The model under review builds one solid part; all positions refer to its coordinate system, in mm. Give positions to 0.01 mm unless a question says otherwise; leave off trailing zeros. Loops run counter-clockwise (first coordinate to the right, second up) from the corner with the lowest first, then second, coordinate; pieces in that order, holes last. Notation, with made-up numbers: M 15,67 L 48,67 A27 cw 48,104 Z; hole C 24,6 d5. An arc over 180 degrees is marked long. Write item = value, one per line. Start each with the question number.
1. For pin 1 (10 mm diameter, centred on y = -126.5, z = 7, fed in from +X); pin 2 (1 mm diameter, centred on y = 130.5, z = 10.5, fed in from +X), all flat-tipped, find the tip position at first contact; note any pin that passes through.
2. We need section A-A on x = -21. Give the boundary of the cut face in (y, z), then the cut area to 3 significant figures.
3. Wall thickness on line 1 along Y through (x, z) = (41, 5); line 2 along X through (y, z) = (125, 12.75); line 3 along X through (y, z) = (146.5, 17.5): over which ranges is each line inside the solid? List them lowest first. Write a range as from..to.
4. We need section C-C on z = 5.75. Give the boundary of the cut face in (x, y).
5. We need section D-D on x = 169. Give the boundary of the cut face in (y, z), then the cut area to 3 significant figures.
6. We need section B-B on y = 136.5. Give the boundary of the cut face in (x, z), then the cut area to 3 significant figures.
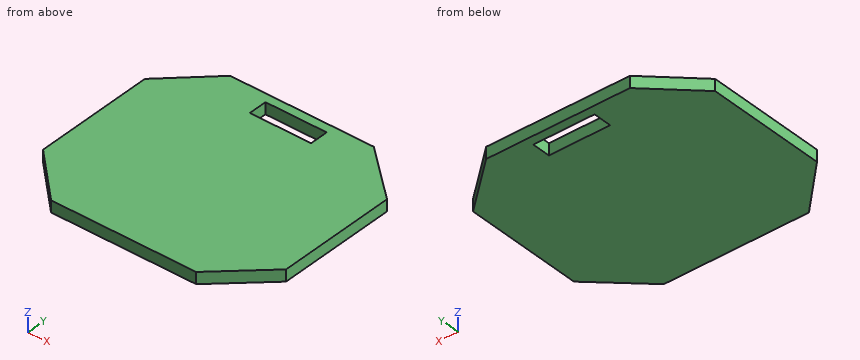
from build123d import *

# Parameters (mm, degrees)
F0_W     = 400
F0_H     = 350
F1_DEPTH = 19
F3_DEPTH = 19.001
F5_DEPTH = 19.001


with BuildPart() as f1:
    # F0 (on Top) → F1 (new body)
    with BuildSketch(Plane.XY):
        Rectangle(F0_W, F0_H)
    extrude(amount=F1_DEPTH)

    # F2 (on face) → F3 (cut, through all)
    with BuildSketch(Plane.XY.offset(19)):
        Polygon((-200, 175), (-200, 100.611582), (-122.030288, 175), align=None)
        Polygon((200, 175), (114.702843, 175), (200, 99.48428), align=None)
        Polygon((200, -97.793318), (116.957434, -175), (200, -175), align=None)
        Polygon((-122.030288, -175), (-200, -98.356977), (-200, -175), align=None)
    extrude(amount=-F3_DEPTH, mode=Mode.SUBTRACT)

    # F4 (on face) → F5 (cut, through all)
    with BuildSketch(Plane.XY.offset(19)):
        Polygon((-51.574003, 160.358503), (-51.574003, 129.921392), (49.319401, 129.921392), (49.319401, 160.358503), (39.737348, 160.358503), align=None)
    extrude(amount=-F5_DEPTH, mode=Mode.SUBTRACT)


solid = f1.part
Final values:
q1.pin_1 = 174.5
q1.pin_2 = 165.53
q2.outline = M -175,0 L 129.92,0 L 129.92,19 L -175,19 Z; M 160.36,0 L 175,0 L 175,19 L 160.36,19 Z
q2.area = 6,070 mm²
q3.line_1 = -175..129.92, 160.36..175
q3.line_2 = -174.44..171.18
q3.line_3 = -151.9..-51.57, 49.32..146.89
q4.outline = M -200,-98.36 L -122.03,-175 L 116.96,-175 L 200,-97.79 L 200,99.48 L 114.7,175 L -122.03,175 L -200,100.61 Z; hole M -51.57,129.92 L 49.32,129.92 L 49.32,160.36 L -51.57,160.36 Z
q5.outline = M -126.61,0 L 126.93,0 L 126.93,19 L -126.61,19 Z
q5.area = 4,820 mm²
q6.outline = M -162.38,0 L -51.57,0 L -51.57,19 L -162.38,19 Z; M 49.32,0 L 158.19,0 L 158.19,19 L 49.32,19 Z
q6.area = 4,170 mm²
